Work out the finished part from the listing and answer in its coordinate system (mm). A direction names the side the tool comes from. Give positions to 0.01 mm unless a question says otherwise; leave off trailing zeros. Order: outer loops, then holes, each group sorted by start corner. A loop starts at its lowest first (then second) coordinate and runs counter-clockwise, first axis right, second up. Notation, with made-up numbers: M -0.75,82.5 L 56.25,82.5 A17 ccw 56.25,104.5 Z; hole C 77.5,57.5 d10. An arc over 180 degrees is marked long. One line per item, written item: value.
from build123d import *

# Parameters (mm, degrees)
SKETCH1_W           = 28.96
SKETCH1_H           = 11
BOSS_EXTRUDE1_DEPTH = 5
SKETCH2_W           = 8.28
SKETCH2_H           = 5
BOSS_EXTRUDE2_DEPTH = 23.1
SKETCH3_W           = 28.96
SKETCH3_H           = 5
BOSS_EXTRUDE3_DEPTH = 8
SKETCH4_W           = 4.56
SKETCH4_H           = 5
CUT_EXTRUDE1_DEPTH  = 5


with BuildPart() as part:
    # Sketch1 → Boss-Extrude1 (new body)
    with BuildSketch(Plane.XY):
        with Locations((-4.078230088, 25.589734513)):
            Rectangle(SKETCH1_W, SKETCH1_H)
    extrude(amount=BOSS_EXTRUDE1_DEPTH)

    # Sketch2 → Boss-Extrude2 (add)
    with BuildSketch(Plane(origin=(0, 31.089734513, 0), x_dir=(1, 0, 0), z_dir=(0, 1, 0))):
        with Locations((-14.418230088, -2.5)):
            Rectangle(SKETCH2_W, SKETCH2_H)
        with Locations((6.261769912, -2.5)):
            Rectangle(SKETCH2_W, SKETCH2_H)
    extrude(amount=BOSS_EXTRUDE2_DEPTH)

    # Sketch3 → Boss-Extrude3 (add)
    with BuildSketch(Plane(origin=(0, 54.189734513, 0), x_dir=(1, 0, 0), z_dir=(0, 1, 0))):
        with Locations((-4.078230088, -2.5)):
            Rectangle(SKETCH3_W, SKETCH3_H)
    extrude(amount=BOSS_EXTRUDE3_DEPTH)

    # Sketch4 → Cut-Extrude1 (cut)
    with BuildSketch(Plane(origin=(0, 31.089734513, 0), x_dir=(1, 0, 0), z_dir=(0, 1, 0))):
        with Locations((-4.078230088, -2.5)):
            Rectangle(SKETCH4_W, SKETCH4_H)
    extrude(amount=-CUT_EXTRUDE1_DEPTH, mode=Mode.SUBTRACT)


solid = part.part
(1) Determine the mould class of faces 3 (the flat face through (-8, 31.09, 2)), 4 (the flat face through (-18.558, 41, 3)), 5 (the flat face through (-1.798, 29, 3)), 6 (the flat face through (-4, 62.19, 2)) for opening direction X: pulls with the +X half, pulls with the -X half, needs draft (parallel to the pull), parting line crosses it, or undercut.
Findings:
face 3: undercut
face 4: pulls with the -X half
face 5: undercut
face 6: needs draft
(2) Section C-C, the plane y = 28 is taken. Give the vertices of the cut face in (x, z), then the cut area to 3 significant figures.
Findings:
outline: M -18.56,0 L -6.36,0 L -6.36,5 L -18.56,5 Z; M -1.8,0 L 10.4,0 L 10.4,5 L -1.8,5 Z
area: 122 mm^2
(3) Section A-A, the plane z = 1.4 is taken. Give the vertices of the cut face in (x, y).
Findings:
outline: M -18.56,20.09 L 10.4,20.09 L 10.4,62.19 L -18.56,62.19 Z; hole M -10.28,31.09 L -6.36,31.09 L -6.36,26.09 L -1.8,26.09 L -1.8,31.09 L 2.12,31.09 L 2.12,54.19 L -10.28,54.19 Z
(4) Given P1, Ø1, axis at x = 0, y = 43.5, coming from the -Z side, flat-ended and moving along its own axis, determine where the tip first touches the part or whether it passes through.
Findings:
P1: passes through
(5) Section B-B, the plane x = -5.25 is taken. Give the vertices of the cut face in (y, z), then the cut area to 3 significant figures.
Findings:
outline: M 20.09,0 L 26.09,0 L 26.09,5 L 20.09,5 Z; M 54.19,0 L 62.19,0 L 62.19,5 L 54.19,5 Z
area: 70.0 mm^2
(6) Which of the six approach directions +Z, -Z, +X, -X, +Y, -Y give full straight-line access (tool end or side, diameter ignored) to faces 1 (the flat face through (-11, 41, 0)), 2 (the flat face through (-6.358, 29, 3))?
Findings:
face 1: -Z, +X, -X, +Y, -Y
face 2: +Z, -Z
(7) Find the intervals of material crossed by probe 1 along X at (y, z) = (39, 0.6); probe 2 along Y at (x, z) = (-6, 2.7); probe 3 along Y at (x, z) = (-6.5, 4.35), in increasing order. Write a range as from..to.
Findings:
probe 1: x = -18.56..-10.28, 2.12..10.4
probe 2: y = 20.09..26.09, 54.19..62.19
probe 3: y = 20.09..31.09, 54.19..62.19
